Verification items for this drawing (mm, ordinates from the low corner). Coordinates: 2 decimals unless noted, no trailing zeros. Write each loop counter-clockwise with the first axis right and the second up, starting at its lowest first coordinate (ties: lowest second). Pieces come first, ordered by that corner, then holes.
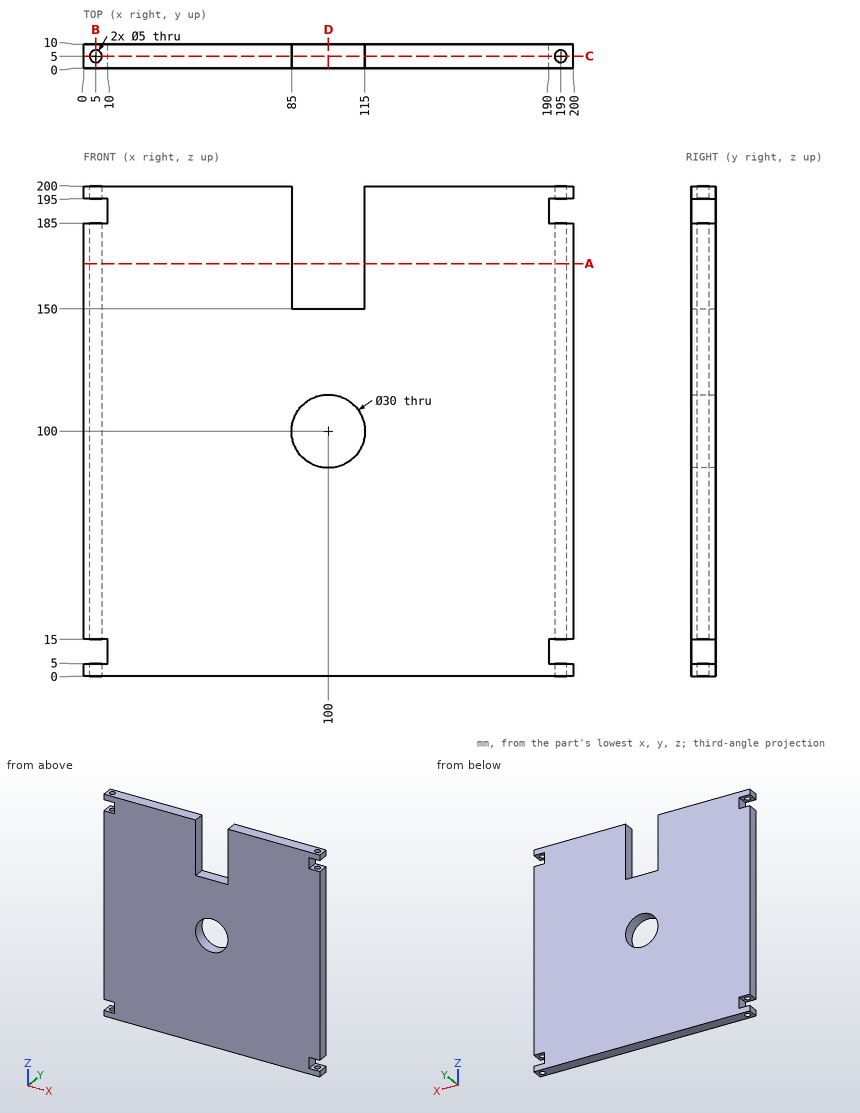
1. Sectioned sample at A-A, the plane z = 168.5. Record the boundary of the cut face in (x, y), and give its area (3 significant figures).
Computed values:
outline: (0, 0) - (85, 0) - (85, 10) - (0, 10) - close; (115, 0) - (200, 0) - (200, 10) - (115, 10) - close; hole circle Ø5 at (5, 5); hole circle Ø5 at (195, 5)
area: 1,660 mm2
2. Sectioned sample at B-B, the plane x = 5. Record the boundary of the cut face in (y, z), and give its area (3 significant figures).
Computed values:
outline: (0, 0) - (2.5, 0) - (2.5, 5) - (0, 5) - close; (0, 15) - (2.5, 15) - (2.5, 185) - (0, 185) - close; (0, 195) - (2.5, 195) - (2.5, 200) - (0, 200) - close; (7.5, 0) - (10, 0) - (10, 5) - (7.5, 5) - close; (7.5, 15) - (10, 15) - (10, 185) - (7.5, 185) - close; (7.5, 195) - (10, 195) - (10, 200) - (7.5, 200) - close
area: 900 mm2
3. Sectioned sample at C-C, the plane y = 5. Give the number of separate pieces and of enclosed holes in the cut face, and give its area (3 significant figures).
Computed values:
separate pieces: 7
enclosed holes: 1
area: 35,600 mm2
4. Sectioned sample at D-D, the plane x = 100. Record the boundary of the cut face in (y, z).
Computed values:
outline: (0, 0) - (10, 0) - (10, 85) - (0, 85) - close; (0, 115) - (10, 115) - (10, 150) - (0, 150) - close
5. Gauge pin test, flat end, axial feed: pin 1 Ø5 at (y, z) = (5.5, 9.5) entering from +X. Record the tip position at first contact, or that the pin passes through.
Computed values:
pin 1: stops at x = 190
6. Thickness scan on line 1 along Y through (x, z) = (195, 196.1); line 2 along X through (y, z) = (1.5, 154.5); line 3 along X through (y, z) = (5.5, 55.5). Record the ranges inside material, lowest first.
Computed values:
line 1: y = 0 to 2.5, 7.5 to 10
line 2: x = 0 to 85, 115 to 200
line 3: x = 0 to 2.55, 7.45 to 192.55, 197.45 to 200
